Geometry check sheet. Reference: the model listing, model coordinates, mm. Round coordinates to 2 decimals unless told otherwise and drop trailing zeros. Loops run counter-clockwise (first coordinate to the right, second up) from the corner with the lowest first, then second, coordinate; pieces in that order, holes last.
```python
from build123d import *

# Parameters (mm, degrees)
SKETCH1_R           = 21
BOSS_EXTRUDE1_DEPTH = 3
SKETCH2_R           = 8
CUT_EXTRUDE1_DEPTH  = 10
CUT_EXTRUDE2_DEPTH  = 10
FILLET1_R           = 3
FILLET2_R           = 1
FILLET3_R           = 3


with BuildPart() as part:
    # Sketch1 → Boss-Extrude1 (new body)
    with BuildSketch(Plane.XY):
        with BuildLine():
            Line((0, 30), (450, 30))
            ThreePointArc((450, 30), (480, 0), (450, -30))
            Line((450, -30), (0, -30))
            ThreePointArc((0, -30), (-30, 0), (0, 30))
        make_face()
        Circle(SKETCH1_R, mode=Mode.SUBTRACT)
    extrude(amount=BOSS_EXTRUDE1_DEPTH)

    # Sketch2 → Cut-Extrude1 (cut)
    with BuildSketch(Plane(origin=(0, 0, 0), x_dir=(-1, 0, 0), z_dir=(0, 0, -1))):
        with Locations((-450, 0)):
            Circle(SKETCH2_R)
    extrude(amount=-CUT_EXTRUDE1_DEPTH, mode=Mode.SUBTRACT)

    # Sketch4 → Cut-Extrude2 (cut)
    with BuildSketch(Plane.XY.offset(3)):
        Polygon((75.051155, 16.751903708), (104.496414244, 16.751903708), (97.010331386, 3.776026753), align=None)
        Polygon((115.236434087, 17.133628969), (159.994947493, 11.590143364), (180.655213039, -0.618195368), (159.994947493, -11.858002091), (118.085145684, -16.966802955), (105.823337098, -0.177570288), align=None)
        Polygon((189.665526052, 18.578346929), (182.941129647, 6.211814834), (165.368544986, 15.767042135), align=None)
        Polygon((199.599828734, 18.578346929), (188.361345274, -0.440625079), (198.44447832, -18.021795356), (236.21688029, -13.651304452), (211.35817569, 15.767042135), align=None)
        Polygon((220.526900823, 17.172694532), (237.960392272, 17.172694532), (260.559362669, 1.057868841), (244.675514904, -10.943884315), align=None)
        Polygon((265.46656767, 6.211814834), (277.833099766, 18.578346929), (248.220353812, 17.874878196), align=None)
        Polygon((165.368544986, -16.358724589), (182.200526719, -6.705265316), (188.690770328, -18.021795356), align=None)
        Polygon((245.637394842, -19.868271823), (269.887796501, -3.220439984), (278.716640894, -18.61460526), align=None)
        Polygon((290.68321902, -21.539751298), (321.940631216, -4.211371592), (335.206376445, -20.70401156), align=None)
        Polygon((341.992933025, 19.183441398), (329.735187473, 1.057868841), (343.614563911, -19.159806148), (373.065049946, 1.057868841), align=None)
        Polygon((273.877820417, 3.11420529), (290.68321902, 20.542728609), (317.209913689, 1.057868841), (284.881711611, -15.886302486), align=None)
        Polygon((305.30736893, 19.270974689), (333.375882047, 18.324324896), (324.94206251, 6.211814834), align=None)
        Polygon((358.198045962, 20.050204211), (388.597492455, 20.050204211), (382.886534474, 8.292807575), align=None)
        Polygon((349.331047186, -24.428108969), (379.030224427, -4.211371592), (391.830023208, -23.92704923), align=None)
        Polygon((386.543005003, -2.048490112), (401.586425759, 20.569577221), (424.881274354, 9.475873595), (434.601030173, -0.440625079), (426.98326683, -8.340846264), (400.664497987, -22.912566492), align=None)
        Polygon((77.908222084, -18.113128875), (99.959146412, -5.986003719), (109.517710051, -19.216558315), align=None)
        Polygon((32.181427401, 14.045195837), (32.181427401, -14.186471438), (52.8225456, -12.955618238), (68.554424875, -10.943884315), (88.302954178, 0), (69.662476286, 10.346921974), (57.571708379, 12.423629667), align=None)
    extrude(amount=-CUT_EXTRUDE2_DEPTH, mode=Mode.SUBTRACT)

    # Fillet1
    # the kernel refuses this fillet: 3 mm, written as the material it adds along each edge
    with BuildSketch(Plane(origin=(32.181427401, 14.045195837, 3), x_dir=(0, -1, 0), z_dir=(0, 0, -1))) as fillet1_piece_1:
        with BuildLine():
            CenterArc((FILLET1_R * 1.06590295895, -FILLET1_R), FILLET1_R, 90, 93.654267812)
            Line((FILLET1_R * 0.0679361503378, -FILLET1_R * 1.06373577423), (0, 0))
            Line((0, 0), (FILLET1_R * 1.06590295895, 0))
        make_face()
    extrude(amount=3)
    with BuildSketch(Plane(origin=(57.571708379, 12.423629667, 3), x_dir=(-0.9979668086083109, 0.06373577422564991, 0), z_dir=(0, 0, -1))) as fillet1_piece_2:
        with BuildLine():
            CenterArc((FILLET1_R * 0.0532106389046, -FILLET1_R), FILLET1_R, 90, 6.091745071)
            Line((-FILLET1_R * 0.0529101714038, -FILLET1_R * 0.00564675611758), (0, 0))
            Line((0, 0), (FILLET1_R * 0.0532106389046, 0))
        make_face()
    extrude(amount=3)
    with BuildSketch(Plane(origin=(69.662476286, 10.346921974, 3), x_dir=(-0.9855678414202016, 0.16928092024302194, 0), z_dir=(0, 0, -1))) as fillet1_piece_3:
        with BuildLine():
            CenterArc((FILLET1_R * 0.169924527084, -FILLET1_R), FILLET1_R, 90, 19.287684891)
            Line((-FILLET1_R * 0.160386998178, -FILLET1_R * 0.0561280297205), (0, 0))
            Line((0, 0), (FILLET1_R * 0.169924527084, 0))
        make_face()
    extrude(amount=3)
    with BuildSketch(Plane(origin=(88.302954178, 0, 3), x_dir=(-0.8743344213622383, 0.48532393266885154, 0), z_dir=(0, 0, -1))) as fillet1_piece_4:
        with BuildLine():
            CenterArc((FILLET1_R * 1.80303637433, -FILLET1_R), FILLET1_R, 90, 121.972748141)
            Line((FILLET1_R * 0.954736326134, -FILLET1_R * 1.52951584323), (0, 0))
            Line((0, 0), (FILLET1_R * 1.80303637433, 0))
        make_face()
    extrude(amount=3)
    with BuildSketch(Plane(origin=(68.554424875, -10.943884315, 3), x_dir=(0.8746742438686059, 0.4847112203290558, 0), z_dir=(0, 0, -1))) as fillet1_piece_5:
        with BuildLine():
            CenterArc((FILLET1_R * 0.191722072286, -FILLET1_R), FILLET1_R, 90, 21.70633324)
            Line((-FILLET1_R * 0.178127385219, -FILLET1_R * 0.0709083044269), (0, 0))
            Line((0, 0), (FILLET1_R * 0.191722072286, 0))
        make_face()
    extrude(amount=3)
    with BuildSketch(Plane(origin=(52.8225456, -12.955618238, 3), x_dir=(0.9919227581955331, 0.1268433749699441, 0), z_dir=(0, 0, -1))) as fillet1_piece_6:
        with BuildLine():
            CenterArc((FILLET1_R * 0.0338255904119, -FILLET1_R), FILLET1_R, 90, 3.874649837)
            Line((-FILLET1_R * 0.0337482743847, -FILLET1_R * 0.00228572587316), (0, 0))
            Line((0, 0), (FILLET1_R * 0.0338255904119, 0))
        make_face()
    extrude(amount=3)
    with BuildSketch(Plane(origin=(32.181427401, -14.186471438, 3), x_dir=(0, 1, 0), z_dir=(0, 0, -1))) as fillet1_piece_7:
        with BuildLine():
            CenterArc((FILLET1_R * 1.06140748795, FILLET1_R), FILLET1_R, 176.587428992, 93.412571008)
            Line((FILLET1_R * 0.0631806961919, FILLET1_R * 1.05952539143), (0, 0))
            Line((0, 0), (FILLET1_R * 1.06140748795, 0))
        make_face()
    extrude(amount=3)

    # Fillet2
    fillet2_edges = [part.edges().sort_by_distance(p)[0] for p in [
        (188.690770328, -18.021795356, 1.5),
        (165.368544986, -16.358724589, 1.5),
        (182.200526719, -6.705265316, 1.5),
        (97.010331386, 3.776026753, 1.5),
        (75.051155, 16.751903708, 1.5),
        (104.496414244, 16.751903708, 1.5),
        (165.368544986, 15.767042135, 1.5),
        (189.665526052, 18.578346929, 1.5),
        (182.941129647, 6.211814834, 1.5),
        (109.517710051, -19.216558315, 1.5),
        (77.908222084, -18.113128875, 1.5),
        (99.959146412, -5.986003719, 1.5),
        (324.94206251, 6.211814834, 1.5),
        (305.30736893, 19.270974689, 1.5),
        (333.375882047, 18.324324896, 1.5),
    ]]
    fillet(fillet2_edges, radius=FILLET2_R)

    # Fillet3
    fillet3_edges = [part.edges().sort_by_distance(p)[0] for p in [
        (199.599828734, 18.578346929, 1.5),
        (211.35817569, 15.767042135, 1.5),
        (236.21688029, -13.651304452, 1.5),
        (198.44447832, -18.021795356, 1.5),
        (188.361345274, -0.440625079, 1.5),
        (400.664497987, -22.912566492, 1.5),
        (386.543005003, -2.048490112, 1.5),
        (401.586425759, 20.569577221, 1.5),
        (424.881274354, 9.475873595, 1.5),
        (434.601030173, -0.440625079, 1.5),
        (426.98326683, -8.340846264, 1.5),
        (341.992933025, 19.183441398, 1.5),
        (373.065049946, 1.057868841, 1.5),
        (343.614563911, -19.159806148, 1.5),
        (329.735187473, 1.057868841, 1.5),
        (284.881711611, -15.886302486, 1.5),
        (273.877820417, 3.11420529, 1.5),
        (290.68321902, 20.542728609, 1.5),
        (317.209913689, 1.057868841, 1.5),
        (244.675514904, -10.943884315, 1.5),
        (220.526900823, 17.172694532, 1.5),
        (237.960392272, 17.172694532, 1.5),
        (260.559362669, 1.057868841, 1.5),
    ]]
    fillet(fillet3_edges, radius=FILLET3_R)


solid = part.part
```
1) Mould release check, pull along X, two halves, no side actions. Record for faces 1 (the face through (87.296, 9.516, 1.521)), 2 (the face through (170.18, 5.57, 1.52)), 3 (the face through (229, 0, 3)), 4 (the face through (-29.993, -0.66, 1.479)): +X half, -X half, draft (parallel to the pull), parting line (faces both ways), or undercut.
Report:
face 1: undercut
face 2: undercut
face 3: draft
face 4: -X half
2) Sectioned sample at B-B, the plane x = 298.5. Record the cut outline in (y, z).
Report:
outline: (-30, 0) - (-21.39, 0) - (-21.39, 3) - (-30, 3) - close; (-17.21, 0) - (-8.75, 0) - (-8.75, 3) - (-17.21, 3) - close; (14.8, 0) - (30, 0) - (30, 3) - (14.8, 3) - close
3) Scan lines: line 1 along Y through (x, z) = (450, 2.3); line 2 along Y through (x, z) = (172, 0.3); line 3 along Y through (x, z) = (383, 2.3). Record each from-to range of solid material in increasing order.
Report:
line 1: y = -30 to -8, 8 to 30
line 2: y = -30 to -16.83, -12.56 to -5.33, 4.5 to 12.16, 16.53 to 30
line 3: y = -30 to -24.03, -10.33 to 8.53, 20.05 to 30
4) Sectioned sample at C-C, the plane z = 1.7. State how many separate pieces and enclosed holes the cut face has, then the cut area to 3 significant figures.
Report:
separate pieces: 1
enclosed holes: 19
area: 18,900 mm2
5) Sectioned sample at A-A, the plane x = 149.5. Record the cut outline in (y, z), then the cut area to 3 significant figures.
Report:
outline: (-30, 0) - (-13.14, 0) - (-13.14, 3) - (-30, 3) - close; (12.89, 0) - (30, 0) - (30, 3) - (12.89, 3) - close
area: 102 mm2
6) Gauge pin test, flat end, axial feed: pin 1 (0.9 mm diameter, centred on y = 4, z = 1.5, fed in from +X). Record the tip position at first contact, or that the pin passes through.
Report:
pin 1: stops at x = 479.79
